Input: part model. Units: mm. Frame: model coordinates. Face numbers are marked on the shaded views. A direction names the side the tool comes from. Coordinates: 2 decimals unless noted, no trailing zeros. Write each loop counter-clockwise with the first axis right and the second up, starting at its lowest first coordinate (ties: lowest second). Pieces come first, ordered by that corner, then holes. Notation, with made-up numbers: (16.25, 20.5) - (64.25, 20.5) arc R8 ccw to (64.25, 32.5) - close; hole circle Ø3 at (-26.5, -33). An arc over 180 degrees is marked (long way). One line per question, with ' | ' between items. Start each with the question number.
1) Line query: line 1 (Z direction, x = 4.75, y = 2.75); line 2 (X direction, y = -4, z = 7); line 3 (X direction, y = -3.75, z = 36.5). Output: solid intervals per line, ascending.
2) Draft query along Z for the marked faces 3, 4, 5 and 6. Return one class per face: released by +Z, released by -Z, zero draft, split by the parting line, or undercut.
3) First-contact query: P1, Ø3, axis at x = -1.5, z = 53, coming from the -Y side; P2, Ø2, axis at y = -4.5, z = 47, coming from the -X side; P3, Ø1.5, axis at x = -0.5, z = 15.5, coming from the +Y side. Flat tips, straight axial feed; report the tip coordinate or a pass-through.
4) Section query A-A on z = 57. Return loops of the section in (x, y).
5) Reachability of the marked faces 1 and 2 from +Z, -Z, +X, -X, +Y, -Y: full face, straight path, thin tool, end or side. Return the list, or none.
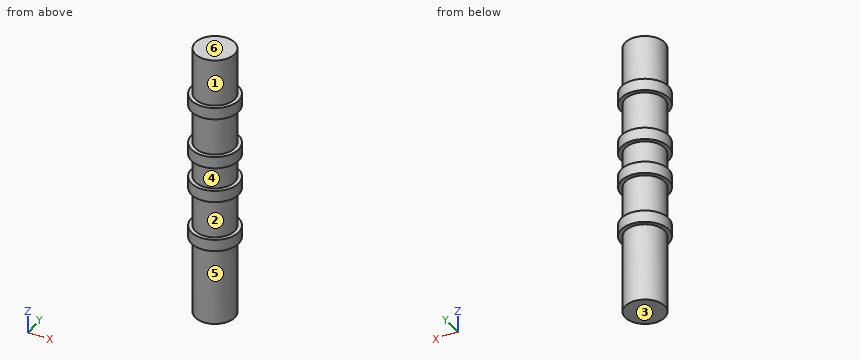
```python
from build123d import *

# Parameters (mm, degrees)
SKETCH1_R           = 5
BOSS_EXTRUDE1_DEPTH = 20
SKETCH2_R           = 6
BOSS_EXTRUDE2_DEPTH = 3
SKETCH3_R           = 5
BOSS_EXTRUDE3_DEPTH = 10
SKETCH4_R           = 6
BOSS_EXTRUDE4_DEPTH = 3
SKETCH5_R           = 5
BOSS_EXTRUDE5_DEPTH = 6
SKETCH6_R           = 6
BOSS_EXTRUDE6_DEPTH = 3
SKETCH7_R           = 5
BOSS_EXTRUDE7_DEPTH = 10
SKETCH8_R           = 6
BOSS_EXTRUDE8_DEPTH = 3
SKETCH9_R           = 5
BOSS_EXTRUDE9_DEPTH = 12


with BuildPart() as part:
    # Sketch1 → Boss-Extrude1 (new body)
    with BuildSketch(Plane.XY):
        Circle(SKETCH1_R)
    extrude(amount=BOSS_EXTRUDE1_DEPTH)

    # Sketch2 → Boss-Extrude2 (add)
    with BuildSketch(Plane.XY.offset(20)):
        Circle(SKETCH2_R)
    extrude(amount=BOSS_EXTRUDE2_DEPTH)

    # Sketch3 → Boss-Extrude3 (add)
    with BuildSketch(Plane.XY.offset(23)):
        Circle(SKETCH3_R)
    extrude(amount=BOSS_EXTRUDE3_DEPTH)

    # Sketch4 → Boss-Extrude4 (add)
    with BuildSketch(Plane.XY.offset(33)):
        Circle(SKETCH4_R)
    extrude(amount=BOSS_EXTRUDE4_DEPTH)

    # Sketch5 → Boss-Extrude5 (add)
    with BuildSketch(Plane.XY.offset(36)):
        Circle(SKETCH5_R)
    extrude(amount=BOSS_EXTRUDE5_DEPTH)

    # Sketch6 → Boss-Extrude6 (add)
    with BuildSketch(Plane.XY.offset(42)):
        Circle(SKETCH6_R)
    extrude(amount=BOSS_EXTRUDE6_DEPTH)

    # Sketch7 → Boss-Extrude7 (add)
    with BuildSketch(Plane.XY.offset(45)):
        Circle(SKETCH7_R)
    extrude(amount=BOSS_EXTRUDE7_DEPTH)

    # Sketch8 → Boss-Extrude8 (add)
    with BuildSketch(Plane.XY.offset(55)):
        Circle(SKETCH8_R)
    extrude(amount=BOSS_EXTRUDE8_DEPTH)

    # Sketch9 → Boss-Extrude9 (add)
    with BuildSketch(Plane.XY.offset(58)):
        Circle(SKETCH9_R)
    extrude(amount=BOSS_EXTRUDE9_DEPTH)


solid = part.part
```
Answer key:
1) line 1: 20 to 23, 33 to 36, 42 to 45, 55 to 58 | line 2: -3 to 3 | line 3: -3.31 to 3.31
2) face 3: released by -Z | face 4: undercut | face 5: zero draft | face 6: released by +Z
3) P1: y = -5 | P2: x = -3.57 | P3: y = 5
4) outline: circle Ø12 at (0, 0)
5) face 1: +Z | face 2: none
